```python
from build123d import *

# Parameters (mm, degrees)
SKETCH1_W                      = 5
SKETCH1_H                      = 110
BOSS_EXTRUDE1_DEPTH            = 120
BOSS_EXTRUDE1_DEPTH_BACK       = 110
BOSS_EXTRUDE1_2_DEPTH          = 120
BOSS_EXTRUDE1_2_DEPTH_BACK     = 110
SKETCH2_W                      = 5
SKETCH2_H                      = 37
BOSS_EXTRUDE2_DEPTH            = 50
SKETCH3_W                      = 220
SKETCH3_H                      = 5
BOSS_EXTRUDE3_DEPTH            = 50
SKETCH4_W                      = 230
SKETCH4_H                      = 73
BOSS_EXTRUDE6_DEPTH            = 5
CUT_EXTRUDE3_DEPTH             = 231
SKETCH5_W                      = 348
SKETCH5_H                      = 227
SKETCH5_W_2                    = 328
SKETCH5_H_2                    = 207
BOSS_EXTRUDE7_DEPTH            = 5
BOSS_EXTRUDE8_DEPTH            = 59
FILLET5_R                      = 15
BOSS_EXTRUDE9_DEPTH            = 5
BOSS_EXTRUDE10_DEPTH           = 5
FILLET6_R                      = 3
CUT_EXTRUDE4_DEPTH             = 165.048773235
SKETCH15_W                     = 45
SKETCH15_H                     = 32
CUT_EXTRUDE5_DEPTH             = 1
CUT_EXTRUDE5_DEPTH_BACK        = 231
SKETCH16_R                     = 1.1
HOLES_FOR_PART_1_DEPTH         = 6
SKETCH17_R                     = 1.1
HOLES_FOR_FORWARD_PART_4_DEPTH = 6
SKETCH18_R                     = 1.1
HOLES_FOR_FORWARD_PART_2_DEPTH = 6
SKETCH19_W                     = 16
SKETCH19_H                     = 60
CUT_EXTRUDE6_DEPTH             = 6


with BuildPart() as part:
    # Sketch1 → Boss-Extrude1 (new body, two sides)
    with BuildSketch(Plane(origin=(0, 0, 0), x_dir=(0, 0, -1), z_dir=(1, 0, 0))) as boss_extrude1_sk:
        with Locations((-112.5, 55)):
            Rectangle(SKETCH1_W, SKETCH1_H)
    extrude(amount=BOSS_EXTRUDE1_DEPTH)
    extrude(boss_extrude1_sk.sketch, amount=-BOSS_EXTRUDE1_DEPTH_BACK)



with BuildPart() as body_2:
    # Sketch1 → Boss-Extrude1 2 (new body, two sides)
    with BuildSketch(Plane(origin=(0, 0, 0), x_dir=(0, 0, -1), z_dir=(1, 0, 0))) as boss_extrude1_2_sk:
        with Locations((112.5, 55)):
            Rectangle(SKETCH1_W, SKETCH1_H)
    extrude(amount=BOSS_EXTRUDE1_2_DEPTH)
    extrude(boss_extrude1_2_sk.sketch, amount=-BOSS_EXTRUDE1_2_DEPTH_BACK)


with BuildPart() as part_1:
    add(part.part)

    add(body_2.part)  # Boss-Extrude2 merges body 2
    # Sketch2 → Boss-Extrude2 (add)
    with BuildSketch(Plane.ZY.offset(110)):
        with Locations((-112.5, 18.5)):
            Rectangle(SKETCH2_W, SKETCH2_H)
        with Locations((112.5, 18.5)):
            Rectangle(SKETCH2_W, SKETCH2_H)
    extrude(amount=BOSS_EXTRUDE2_DEPTH)

    # Sketch3 → Boss-Extrude3 (add)
    with BuildSketch(Plane.ZY.offset(160)):
        with Locations((0, 34.5)):
            Rectangle(SKETCH3_W, SKETCH3_H)
    extrude(amount=-BOSS_EXTRUDE3_DEPTH)

    # Sketch4 → Boss-Extrude6 (add)
    with BuildSketch(Plane.ZY.offset(110)):
        with Locations((0, 73.5)):
            Rectangle(SKETCH4_W, SKETCH4_H)
    extrude(amount=BOSS_EXTRUDE6_DEPTH)

    # Sketch9 → Cut-Extrude3 (cut, through all)
    with BuildSketch(Plane.XY.offset(115)):
        Polygon((120, 110), (116.464466094, 106.464466094), (120, 102.928932188), align=None)
    extrude(amount=-CUT_EXTRUDE3_DEPTH, mode=Mode.SUBTRACT)

    # Sketch10 → Boss-Extrude8 (add)
    with BuildSketch(Plane.XY.offset(115)):
        Polygon((120, 110), (111.464466094, 110), (111.464466094, 0), (120, 0), (120, 102.928932188), (116.464466094, 106.464466094), align=None)
    boss_extrude8 = extrude(amount=BOSS_EXTRUDE8_DEPTH)

    # Mirror3: Boss-Extrude8 across plane
    add(boss_extrude8.mirror(Plane.XY))

    # Fillet5
    fillet5_edges = [part_1.edges().sort_by_distance(p)[0] for p in [
        (111.464466094, 55, 115),
        (111.464466094, 55, -115),
    ]]
    fillet(fillet5_edges, radius=FILLET5_R)

    # Fillet6
    fillet6_edges = [part_1.edges().sort_by_distance(p)[0] for p in [
        (111.464466094, 55, 174),
        (111.464466094, 55, -174),
    ]]
    fillet(fillet6_edges, radius=FILLET6_R)


with BuildPart() as body_2_2:
    # Sketch5 → Boss-Extrude7 (new body)
    with BuildSketch(Plane(origin=(115, 115, 0), x_dir=(0, 0, 1), z_dir=(-0.707106781, -0.707106781, 0))):
        with Locations((0, -120.571067812)):
            Rectangle(SKETCH5_W, SKETCH5_H)
        with Locations((0, -120.571067812)):
            Rectangle(SKETCH5_W_2, SKETCH5_H_2, mode=Mode.SUBTRACT)
    extrude(amount=BOSS_EXTRUDE7_DEPTH)


with BuildPart() as body_3:
    # Sketch12 → Boss-Extrude9 (new body)
    with BuildSketch(Plane.XY.offset(174)):
        Polygon((120, 0), (222.928932188, 0), (120, 102.928932188), align=None)
    extrude(amount=-BOSS_EXTRUDE9_DEPTH)


with BuildPart() as body_4:
    # Sketch13 → Boss-Extrude10 (new body)
    with BuildSketch(Plane(origin=(0, 0, -174), x_dir=(-1, 0, 0), z_dir=(0, 0, -1))):
        Polygon((-120, 102.928932188), (-120, 0), (-222.928932188, 0), align=None)
    extrude(amount=-BOSS_EXTRUDE10_DEPTH)


with BuildPart() as cut_extrude4_tool:
    # Sketch14 → Cut-Extrude4 (new body, through all)
    with BuildSketch(Plane(origin=(0, 110, 0), x_dir=(1, 0, 0), z_dir=(0, 1, 0))):
        Polygon((-115, 115), (-115, -115), (-167.30995795, -115), (-167.30995795, -200.602059027), (289.684331767, -200.602059027), (289.684331767, -115), (289.684331767, 105), (289.684331767, 193.761157723), (-167.30995795, 193.761157723), (-167.30995795, 115), align=None)
    extrude(amount=-CUT_EXTRUDE4_DEPTH)


with BuildPart() as part_2:
    add(part_1.part)

    # Cut-Extrude4: cut by cut_extrude4_tool
    add(cut_extrude4_tool.part, mode=Mode.SUBTRACT)

    # Sketch15 → Cut-Extrude5 (cut, two sides)
    with BuildSketch(Plane.XY.offset(115)) as cut_extrude5_sk:
        with Locations((-137.5, 16)):
            Rectangle(SKETCH15_W, SKETCH15_H)
    extrude(amount=CUT_EXTRUDE5_DEPTH, mode=Mode.SUBTRACT)
    extrude(cut_extrude5_sk.sketch, amount=-CUT_EXTRUDE5_DEPTH_BACK, mode=Mode.SUBTRACT)

    # Sketch16 → Holes for part 1 (cut, through all)
    with BuildSketch(Plane(origin=(0, 37, 0), x_dir=(1, 0, 0), z_dir=(0, 1, 0))):
        with Locations((-150, -100)):
            Circle(SKETCH16_R)
        with Locations((-150, -90)):
            Circle(SKETCH16_R)
        with Locations((-150, 90)):
            Circle(SKETCH16_R)
        with Locations((-150, 100)):
            Circle(SKETCH16_R)
    extrude(amount=-HOLES_FOR_PART_1_DEPTH, mode=Mode.SUBTRACT)

    # Sketch17 → Holes for forward part 4 (cut, through all)
    with BuildSketch(Plane(origin=(0, 37, 0), x_dir=(1, 0, 0), z_dir=(0, 1, 0))):
        with Locations((-121, 70)):
            Circle(SKETCH17_R)
        with Locations((-121, -70)):
            Circle(SKETCH17_R)
    extrude(amount=-HOLES_FOR_FORWARD_PART_4_DEPTH, mode=Mode.SUBTRACT)

    # Sketch18 → Holes for forward part 2 (cut, through all)
    with BuildSketch(Plane(origin=(0, 37, 0), x_dir=(1, 0, 0), z_dir=(0, 1, 0))):
        with Locations((-134, 50)):
            Circle(SKETCH18_R)
        with Locations((-144, 50)):
            Circle(SKETCH18_R)
        with Locations((-144, -50)):
            Circle(SKETCH18_R)
        with Locations((-134, -50)):
            Circle(SKETCH18_R)
    extrude(amount=-HOLES_FOR_FORWARD_PART_2_DEPTH, mode=Mode.SUBTRACT)

    # Sketch19 → Cut-Extrude6 (cut, through all)
    with BuildSketch(Plane(origin=(0, 37, 0), x_dir=(1, 0, 0), z_dir=(0, 1, 0))):
        with Locations((-160, 0)):
            Rectangle(SKETCH19_W, SKETCH19_H)
    extrude(amount=-CUT_EXTRUDE6_DEPTH, mode=Mode.SUBTRACT)


with BuildPart() as body_2_2_1:
    add(body_2_2.part)

    # Cut-Extrude4: cut by cut_extrude4_tool
    add(cut_extrude4_tool.part, mode=Mode.SUBTRACT)


with BuildPart() as body_3_1:
    add(body_3.part)

    # Cut-Extrude4: cut by cut_extrude4_tool
    add(cut_extrude4_tool.part, mode=Mode.SUBTRACT)


with BuildPart() as body_4_1:
    add(body_4.part)

    # Cut-Extrude4: cut by cut_extrude4_tool
    add(cut_extrude4_tool.part, mode=Mode.SUBTRACT)


solid = part_2.part
```
Source: CAD feature listing. Evaluate the final solid. Frame: model axes, mm. A direction names the side the tool comes from. Round coordinates to 2 decimals unless told otherwise and drop trailing zeros. Use a Markdown table: item, result. Add a question column.
1. Section query A-A on y = 35.1. Give the number of separate pieces and of enclosed holes in the cut face, then the cut area to 3 significant figures.
2. Reachability of faces 4 (the flat face through (-156, 35, -30)), 5 (the flat face through (-115, 35, -2)) from +Z, -Z, +X, -X, +Y, -Y: full face, straight path, thin tool, end or side. Return the list, or none.
3. Mould query, pull axis Z, two halves, no side actions, for faces 1 (the flat face through (-152, 35, 0)), 2 (the flat face through (-138, 32, 2)), 3 (the flat face through (-137, 34, 115)). Classes: pulls with the +Z half, pulls with the -Z half, needs draft (parallel to the pull), parting line crosses it, or undercut.
4. Line query: line 1 (Z direction, x = -153.5, y = 33.05); line 2 (Z direction, x = -134, y = 35.15); line 3 (X direction, y = 34.3, z = -50). Output: solid intervals per line, ascending.
5. Contact query for a flat-ended pin moving along its axis: P1, Ø2, axis at x = -134, z = 50, coming from the +Y side. Output: stop coordinate, or through.
Reported:
| question | item | result |
|---|---|---|
| 1 | separate pieces | 1 |
| 1 | enclosed holes | 10 |
| 1 | area | 9,830 mm² |
| 2 | face 4 | -X, +Y, -Y |
| 2 | face 5 | +Z, -Z, +X, +Y, -Y |
| 3 | face 1 | undercut |
| 3 | face 2 | needs draft |
| 3 | face 3 | pulls with the +Z half |
| 4 | line 1 | z = -115 to -30, 30 to 115 |
| 4 | line 2 | z = -115 to -51.1, -48.9 to 48.9, 51.1 to 115 |
| 4 | line 3 | x = -160 to -145.1, -142.9 to -135.1, -132.9 to -115 |
| 5 | P1 | passes through |
